from build123d import *

# Parameters (mm, degrees)
SKETCH_1_W          = 14
SKETCH_1_H          = 14
SKETCH_1_W_2        = 12
SKETCH_1_H_2        = 12
EXTRUDE_1_DEPTH     = 7
SKETCH_2_W          = 3
SKETCH_2_H          = 7
EXTRUDE_2_DEPTH     = 3.5
SKETCH_3_R          = 0.75
CUT_EXTRUDE_1_DEPTH = 15.43086969
CUT_EXTRUDE_2_DEPTH = 15.43086969


with BuildPart() as part:
    # 草图1 → 凸台-拉伸1 (new body)
    with BuildSketch(Plane.XY):
        Rectangle(SKETCH_1_W, SKETCH_1_H)
        Rectangle(SKETCH_1_W_2, SKETCH_1_H_2, mode=Mode.SUBTRACT)
    extrude(amount=EXTRUDE_1_DEPTH)

    # 草图2 → 凸台-拉伸2 (add)
    with BuildSketch(Plane.XZ.offset(7)):
        with Locations((0, 3.5)):
            Rectangle(SKETCH_2_W, SKETCH_2_H)
    extrude_2 = extrude(amount=EXTRUDE_2_DEPTH)

    # 草图3 → 切除-拉伸1 (cut, through all)
    with BuildSketch(Plane.XY.offset(7)):
        with Locations((0, -9)):
            Circle(SKETCH_3_R)
    cut_extrude_1 = extrude(amount=-CUT_EXTRUDE_1_DEPTH, mode=Mode.SUBTRACT)

    # 草图3<3> → 切除-拉伸2 (cut, through all)
    with BuildSketch(Plane.XY.offset(7)):
        with BuildLine():
            ThreePointArc((0, -10.5), (-1.060660172, -10.060660172), (-1.5, -9))
            Line((-1.5, -9), (-1.5, -10.5))
            Line((-1.5, -10.5), (0, -10.5))
        make_face()
        with BuildLine():
            Line((1.5, -10.5), (1.5, -9))
            ThreePointArc((1.5, -9), (1.060660172, -10.060660172), (0, -10.5))
            Line((0, -10.5), (1.5, -10.5))
        make_face()
    cut_extrude_2 = extrude(amount=-CUT_EXTRUDE_2_DEPTH, mode=Mode.SUBTRACT)

    # 镜向1: 凸台-拉伸2, 切除-拉伸1, 切除-拉伸2 across plane
    add(extrude_2.mirror(Plane.ZX))
    add(cut_extrude_1.mirror(Plane.ZX), mode=Mode.SUBTRACT)
    add(cut_extrude_2.mirror(Plane.ZX), mode=Mode.SUBTRACT)


solid = part.part
Read the model definition and answer for the solid it produces. Units are mm, in the model's axes. A direction names the side the tool comes from. Coordinates: 2 decimals unless noted, no trailing zeros. Write each loop counter-clockwise with the first axis right and the second up, starting at its lowest first coordinate (ties: lowest second). Pieces come first, ordered by that corner, then holes. Notation, with made-up numbers: (27.25, 44) - (31.25, 44) arc R12 ccw to (31.25, 54) - close; hole circle Ø2 at (13.25, -14.75). An arc over 180 degrees is marked (long way). One line per question, with ' | ' between items.
Q1. Find section C-C, the plane z = 3.75. Write down the section's boundary in (x, y), plus the area to 3 significant figures.
Result set:
outline: (-7, -7) - (-1.5, -7) - (-1.5, -9) arc R1.5 ccw to (1.5, -9) - (1.5, -7) - (7, -7) - (7, 7) - (1.5, 7) - (1.5, 9) arc R1.5 ccw to (-1.5, 9) - (-1.5, 7) - (-7, 7) - close; hole (-6, -6) - (6, -6) - (6, 6) - (-6, 6) - close; hole circle Ø1.5 at (0, -9); hole circle Ø1.5 at (0, 9) | area: 67.5 mm^2
Q2. Determine the mould class of faces 5 (the flat face through (1.5, -8, 3)), 6 (the flat face through (-7, 0, 3)), 7 (the flat face through (0, 6, 3)) for opening direction X: +X half, -X half, draft (parallel to the pull), parting line (faces both ways), or undercut.
Result set:
face 5: +X half | face 6: -X half | face 7: undercut
Q3. For faces 1 (the flat face through (-1.5, 8, 3)), 2 (the flat face through (4, -7, 3)), 3 (the flat face through (-4, -7, 3)), 4 (the flat face through (-6, 0, 3)), determine the directions among +Z, -Z, +X, -X, +Y, -Y from which every point of the face is accessible in a straight line to the end or side of a thin tool.
Result set:
face 1: +Z, -Z, -X, +Y | face 2: +Z, -Z, +X, -Y | face 3: +Z, -Z, -X, -Y | face 4: +Z, -Z
Q4. Find section A-A, the plane y = -0.5. Write down the section's boundary in (x, z).
Result set:
outline: (-7, 0) - (-6, 0) - (-6, 7) - (-7, 7) - close; (6, 0) - (7, 0) - (7, 7) - (6, 7) - close
Q5. Consider L1, parallel to Y at x = 0, z = 2.5; L2, parallel to Y at x = -2.75, z = 2. Determine where each line is inside the solid, lowest interval first. Write a range as [from, to].
Result set:
L1: [-10.5, -9.75], [-8.25, -6], [6, 8.25], [9.75, 10.5] | L2: [-7, -6], [6, 7]
Q6. Each of these flat-tipped pins is pushed along its axis until it touches: P1, Ø1, axis at y = -8.5, z = 3, coming from the +X side; P2, Ø3, axis at x = -5.5, z = 4, coming from the -Y side; P3, Ø2, axis at x = -1.5, z = 3, coming from the -Y side. Where does it stop, or does it pass through?
Result set:
P1: x = 1.5 | P2: y = -7 | P3: y = -10.41
Q7. Find section D-D, the plane y = -8. Write down the section's boundary in (x, z).
Result set:
outline: (-1.5, 0) - (1.5, 0) - (1.5, 7) - (-1.5, 7) - close
